Read the model definition and answer for the solid it produces. Units are mm, in the model's axes. Coordinates: 2 decimals unless noted, no trailing zeros. Order: outer loops, then holes, each group sorted by start corner. A loop starts at its lowest first (then second) coordinate and runs counter-clockwise, first axis right, second up. Notation, with made-up numbers: (33, -23) - (88, -23) arc R15 ccw to (88, -2) - close; hole circle Ø1 at (-24, -8). An arc over 180 degrees is marked (long way). Use one line per item in the form item = value.
```python
from build123d import *

# Parameters (mm, degrees)
BOSS_EXTRUDE1_DEPTH = 85
SKETCH3_R           = 2.15
CUT_EXTRUDE1_DEPTH  = 85
LPATTERN1_COUNT     = 4
LPATTERN1_PITCH     = 15
SKETCH4_R           = 2.15
CUT_EXTRUDE2_DEPTH  = 85


with BuildPart() as part:
    # Sketch2 → Boss-Extrude1 (new body)
    with BuildSketch(Plane.XY):
        Polygon((0, 0), (96.674271247, 0), (92.532135624, 10), (4.142135624, 10), align=None)
    extrude(amount=BOSS_EXTRUDE1_DEPTH)

    # Sketch3 → Cut-Extrude1 (cut)
    with BuildSketch(Plane.XZ):
        with Locations(Location((25, 75, 0), (0, 0, 270))):
            Circle(SKETCH3_R)
        with Locations((25, 10)):
            Circle(SKETCH3_R)
    cut_extrude1 = extrude(amount=-CUT_EXTRUDE1_DEPTH, mode=Mode.SUBTRACT)

    # LPattern1: Cut-Extrude1 ×4
    with Locations(*[(i * LPATTERN1_PITCH, 0, 0) for i in range(1, LPATTERN1_COUNT)]):
        add(cut_extrude1, mode=Mode.SUBTRACT)

    # Sketch4 → Cut-Extrude2 (cut)
    with BuildSketch(Plane(origin=(0, 10, 0), x_dir=(1, 0, 0), z_dir=(0, 1, 0))):
        with Locations(Location((83.532135624, -20, 0), (0, 0, 180))):
            Circle(SKETCH4_R)
        with Locations(Location((83.532135624, -42.5, 0), (0, 0, 180))):
            Circle(SKETCH4_R)
        with Locations(Location((83.532135624, -65, 0), (0, 0, 180))):
            Circle(SKETCH4_R)
        with Locations(Location((13.142135624, -65, 0), (0, 0, 270))):
            Circle(SKETCH4_R)
        with Locations(Location((13.142135624, -42.5, 0), (0, 0, 270))):
            Circle(SKETCH4_R)
        with Locations(Location((13.142135624, -20, 0), (0, 0, 270))):
            Circle(SKETCH4_R)
    extrude(amount=-CUT_EXTRUDE2_DEPTH, mode=Mode.SUBTRACT)


solid = part.part
```
(1) Given pin 1 Ø5 at (x, z) = (70, 75) entering from -Y; pin 2 Ø4 at (y, z) = (4.5, 17.5) entering from -X; pin 3 Ø1 at (y, z) = (4.5, 66.5) entering from -X, each flat-ended and moving along its own axis, determine where each tip first touches the part or whether it passes through.
Answer list:
pin_1 = 0
pin_2 = 1.04
pin_3 = 1.66
(2) Section C-C, the plane z = 42.5 is taken. Write down the section's boundary in (x, y), then the cut area to 3 significant figures.
Answer list:
outline = (0, 0) - (10.99, 0) - (10.99, 10) - (4.14, 10) - close; (15.29, 0) - (81.38, 0) - (81.38, 10) - (15.29, 10) - close; (85.68, 0) - (96.67, 0) - (92.53, 10) - (85.68, 10) - close
area = 839 mm2
(3) Section A-A, the plane x = 25 is taken. Write down the section's boundary in (y, z), then the cut area to 3 significant figures.
Answer list:
outline = (0, 0) - (10, 0) - (10, 7.85) - (0, 7.85) - close; (0, 12.15) - (10, 12.15) - (10, 72.85) - (0, 72.85) - close; (0, 77.15) - (10, 77.15) - (10, 85) - (0, 85) - close
area = 764 mm2
(4) Section D-D, the plane y = 8.75 is taken. State how many separate pieces and enclosed holes the cut face has, then the cut area to 3 significant figures.
Answer list:
separate_pieces = 1
enclosed_holes = 14
area = 7,400 mm2
(5) The mould has two halves that part along Z. Classify faces 1 (the flat face through (94.632, 4.93, 41.905)), 2 (the flat face through (48, 5, 85)), 3 (the cylindrical face through (68.294, 4.93, 8.692)): +Z half, -Z half, draft (parallel to the pull), parting line (faces both ways), or undercut.
Answer list:
face_1 = draft
face_2 = +Z half
face_3 = undercut
(6) Straight lines are drawn through the part: L1, parallel to Z at x = 54.5, y = 6.75; L2, parallel to X at y = 5.25, z = 75; L3, parallel to Z at x = 84.5, y = 6.5. For each, find the intervals that lie inside material, in ascending order.
Answer list:
L1 = 0 to 7.91, 12.09 to 72.91, 77.09 to 85
L2 = 2.17 to 22.85, 27.15 to 37.85, 42.15 to 52.85, 57.15 to 67.85, 72.15 to 94.5
L3 = 0 to 18.08, 21.92 to 40.58, 44.42 to 63.08, 66.92 to 85
(7) Section B-B, the plane z = 10 is taken. Write down the section's boundary in (x, y).
Answer list:
outline = (0, 0) - (22.85, 0) - (22.85, 10) - (4.14, 10) - close; (27.15, 0) - (37.85, 0) - (37.85, 10) - (27.15, 10) - close; (42.15, 0) - (52.85, 0) - (52.85, 10) - (42.15, 10) - close; (57.15, 0) - (67.85, 0) - (67.85, 10) - (57.15, 10) - close; (72.15, 0) - (96.67, 0) - (92.53, 10) - (72.15, 10) - close
